Verification items for the finished model (mm, model axes). Coordinates: 2 decimals unless noted, no trailing zeros. Loops run counter-clockwise (first coordinate to the right, second up) from the corner with the lowest first, then second, coordinate; pieces in that order, holes last.
Q1. Material ranges on probe 1 along Y at (x, z) = (7.5, 0.7); probe 2 along X at (y, z) = (17.5, 0.4); probe 3 along X at (y, z) = (8.5, 0.7), recorded low to high.
Q2. Sectioned sample at B-B (y = 33.5). Enter the section's corners in (x, z), then the cut area to 3 significant figures.
Q3. Sectioned sample at A-A (z = 0.4). Enter the section's corners in (x, y) (1 decimal).
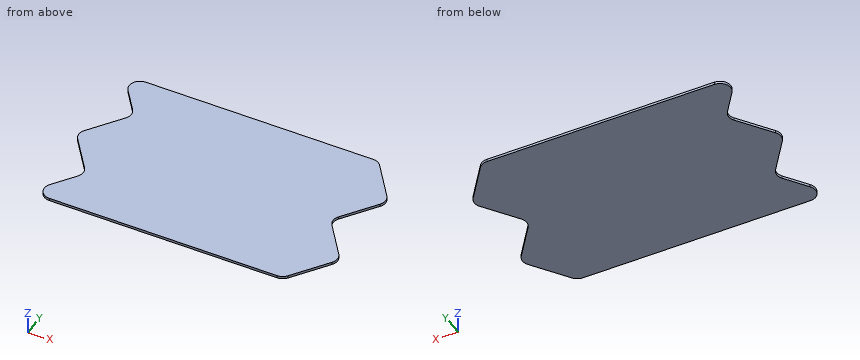
```python
from build123d import *

# Parameters (mm, degrees)
F1_DEPTH = 0.76
F2_R     = 3.18


with BuildPart() as f1:
    # F0 (on Top) → F1 (new body)
    with BuildSketch(Plane.XY):
        Polygon((85.6, 40.485), (75.6, 53.98), (0, 53.98), (10, 40.485), (0, 26.99), (10, 13.495), (0, 0), (75.6, 0), (85.6, 13.495), (75.6, 26.99), align=None)
    extrude(amount=F1_DEPTH)

    # F2
    f2_edges = [f1.edges().sort_by_distance(p)[0] for p in [
        (0, 53.98, 0.38),
        (10, 40.485, 0.38),
        (0, 26.99, 0.38),
        (10, 13.495, 0.38),
        (0, 0, 0.38),
        (75.6, 53.98, 0.38),
        (85.6, 40.485, 0.38),
        (75.6, 26.99, 0.38),
        (85.6, 13.495, 0.38),
        (75.6, 0, 0.38),
    ]]
    fillet(f2_edges, radius=F2_R)


solid = f1.part
```
Geometry check:
1. probe 1: y = 0 to 10.12, 16.87 to 37.11, 43.86 to 53.98
1. probe 2: x = 7.03 to 82.63
1. probe 3: x = 6.3 to 81.9
2. outline: (4.82, 0) - (80.42, 0) - (80.42, 0.76) - (4.82, 0.76) - close
2. area: 57.5 mm2
3. outline: (1.4, 25.1) - (8.6, 15.4) arc R3.2 cw to (8.6, 11.6) - (3.8, 5.1) arc R3.2 ccw to (6.3, 0) - (74, 0) arc R3.2 ccw to (76.6, 1.3) - (84.2, 11.6) arc R3.2 ccw to (84.2, 15.4) - (77, 25.1) arc R3.2 cw to (77, 28.9) - (84.2, 38.6) arc R3.2 ccw to (84.2, 42.4) - (76.6, 52.7) arc R3.2 ccw to (74, 54) - (6.3, 54) arc R3.2 ccw to (3.8, 48.9) - (8.6, 42.4) arc R3.2 cw to (8.6, 38.6) - (1.4, 28.9) arc R3.2 ccw to start
